Part print with two shaded views. Sizes in mm from the minimum x, y, z corner. A direction names the side the tool comes from. Give positions to 0.01 mm unless a question says otherwise; leave off trailing zeros. Write each loop counter-clockwise with the first axis right and the second up, starting at its lowest first coordinate (ties: lowest second). Pieces come first, ordered by that corner, then holes. Notation, with made-up numbers: (41.5, -15.75) - (48.5, -15.75) arc R28 cw to (48.5, 3.25) - close; hole circle Ø6 at (-28.5, -6). An arc over 180 degrees is marked (long way). One line per item, written item: value. Start each with the question number.
(1) 3-axis set-ups, long thin cutter, end or side, ignore diameter. For the marked faces 4, 5 and 6: which of +Z, -Z, +X, -X, +Y, -Y reach the whole face in a straight line?
(2) Probe L1, parallel to X at y = 4, z = 5 (1 decimal); L2, parallel to X at y = 87.5, z = 20; L3, parallel to Y at x = 71.5, z = 4 (1 decimal). List the from-to ranges inside material, lowest first.
(3) Mould opens along X. For the marked faces 1, 2 and 3 say: pulls with the +X half, pulls with the -X half, needs draft (parallel to the pull), parting line crosses it, or undercut.
(4) Drop flat-ended pins along their axis: P1, Ø1, axis at x = 51, z = 20.5, coming from the +Y side; P2, Ø5.5, axis at x = 6.8, y = 95.5, coming from the +Z side. Give the stop position or say it passes through.
(5) Cut at B-B, the plane x = 44. List the corners of the cut face in (y, z).
(6) Cut at C-C, the plane y = 91. List the corners of the cut face in (x, z).
(7) Cut at A-A, the plane z = 16. List the corners of the cut face in (x, y), and give its area (3 significant figures).
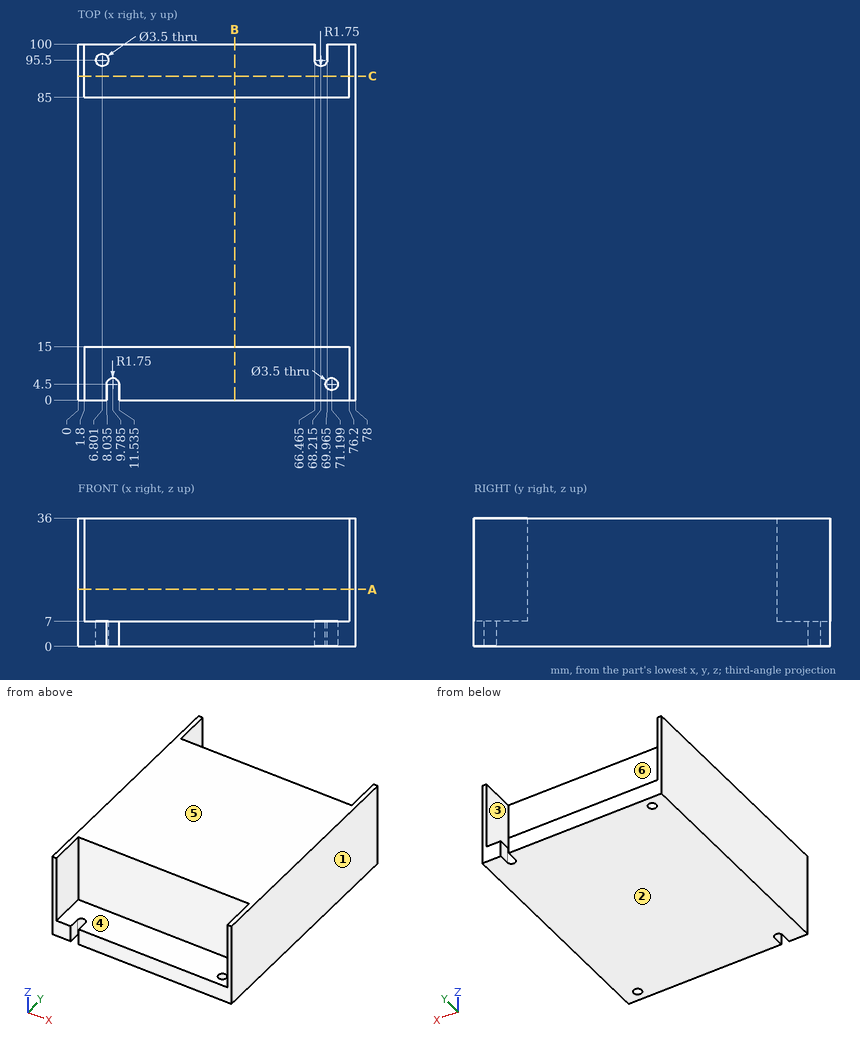
Answers follow:
1. face 4: +Z, -Y
1. face 5: +Z, +X, -X, +Y, -Y
1. face 6: +Z, +Y
2. L1: x = 0 to 8, 11.5 to 69.5, 72.9 to 78
2. L2: x = 0 to 1.8, 76.2 to 78
2. L3: y = 0 to 2.8, 6.2 to 100
3. face 1: pulls with the +X half
3. face 2: needs draft
3. face 3: undercut
4. P1: stops at y = 85
4. P2: stops at z = 7
5. outline: (0, 0) - (100, 0) - (100, 7) - (85, 7) - (85, 36) - (15, 36) - (15, 7) - (0, 7) - close
6. outline: (0, 0) - (78, 0) - (78, 36) - (76.2, 36) - (76.2, 7) - (1.8, 7) - (1.8, 36) - (0, 36) - close
7. outline: (0, 0) - (1.8, 0) - (1.8, 15) - (76.2, 15) - (76.2, 0) - (78, 0) - (78, 100) - (76.2, 100) - (76.2, 85) - (1.8, 85) - (1.8, 100) - (0, 100) - close
7. area: 5,570 mm²
